Build history of the part. All positions in model axes, mm. Face numbers are marked on the shaded views. A direction names the side the tool comes from. Coordinates: 2 decimals unless noted, no trailing zeros. Order: outer loops, then holes, each group sorted by start corner. A loop starts at its lowest first (then second) coordinate and runs counter-clockwise, first axis right, second up. Notation, with made-up numbers: M 67.25,-35 L 120.25,-35 A23 cw 120.25,-21 Z; hole C -13.5,21 d11. An arc over 180 degrees is marked long. Write item = value, one per line. Start each with the question number.
Q1. Band-saw the part on D-D on z = 11.25. Write the cut outline in (x, y).
Q2. Band-saw the part on C-C on x = -4. Write the cut outline in (y, z).
Q3. Drill centre lines: probe 1 along Y at (x, z) = (-4, 0.6); probe 2 along Z at (x, y) = (2.5, 13); probe 3 along Y at (x, z) = (7, 15.5). Where is each one in solid material? Low to high.
Q4. Pin check, flat tips, straight feed: P1, Ø5, axis at x = -13, z = 17, coming from the +Y side; P2, Ø12, axis at x = 13.5, y = 10, coming from the +Z side. Stop position of each tip, or through.
Q5. Band-saw the part on A-A on y = -1.75. Write the cut outline in (x, z).
Q6. Band-saw the part on B-B on y = -12.75. Write the cut outline in (x, z).
Q7. 3-axis set-ups, long thin cutter, end or side, ignore diameter. For the marked faces 1 and 2: which of +Z, -Z, +X, -X, +Y, -Y reach the whole face in a straight line?
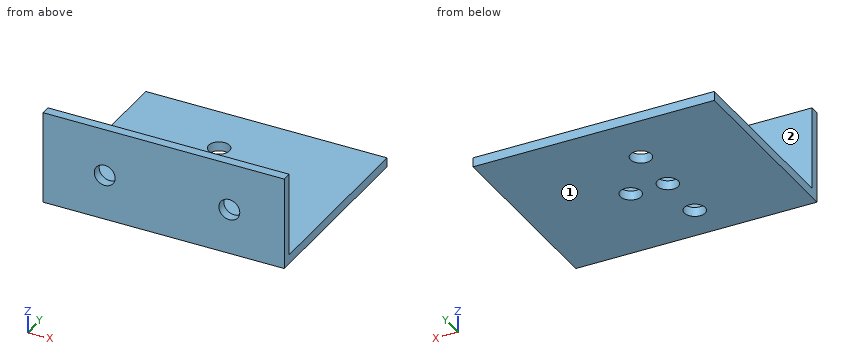
```python
from build123d import *

# Parameters (mm, degrees)
ESQUISSE1_W             = 52
ESQUISSE1_H             = 42
BOSS_EXTRU_1_DEPTH      = 20
ESQUISSE2_W             = 66.008627658
ESQUISSE2_H             = 40.946179855
ENL_V_MAT_EXTRU_1_DEPTH = 40
D_GAGEMENT_M41_D        = 4.5
D_GAGEMENT_M42_D        = 4.5


with BuildPart() as part:
    # Esquisse1 → Boss.-Extru.1 (new body)
    with BuildSketch(Plane.XY):
        Rectangle(ESQUISSE1_W, ESQUISSE1_H)
    extrude(amount=BOSS_EXTRU_1_DEPTH)

    # Esquisse2 → Enlèv. mat.-Extru.1 (cut)
    with BuildSketch(Plane(origin=(0, 21, 0), x_dir=(1, 0, 0), z_dir=(0, 1, 0))):
        with Locations((1.405901571, -22.473089928)):
            Rectangle(ESQUISSE2_W, ESQUISSE2_H)
    extrude(amount=-ENL_V_MAT_EXTRU_1_DEPTH, mode=Mode.SUBTRACT)

    # Dégagement M41 (through all)
    with Locations(Plane(origin=(0, 0, 0), x_dir=(-1, 0, 0), z_dir=(0, 0, -1))):
        with Locations((4, -12.75), (4, -1.75), (4, 9.25), (-4, -1.75)):
            Hole(D_GAGEMENT_M41_D / 2)

    # Dégagement M42 (through all)
    with Locations(Plane(origin=(0, -19, 0), x_dir=(1, 0, 0), z_dir=(0, 1, 0))):
        with Locations((-12.695679618, -9.785063319), (14.163037838, -9.785063319)):
            Hole(D_GAGEMENT_M42_D / 2)


solid = part.part
```
Recorded:
q1.outline = M -26,-21 L -14.4,-21 L -14.4,-19 L -26,-19 Z; M -10.99,-21 L 12.46,-21 L 12.46,-19 L -10.99,-19 Z; M 15.87,-21 L 26,-21 L 26,-19 L 15.87,-19 Z
q2.outline = M -21,0 L -15,0 L -15,2 L -19,2 L -19,20 L -21,20 Z; M -10.5,0 L -4,0 L -4,2 L -10.5,2 Z; M 0.5,0 L 7,0 L 7,2 L 0.5,2 Z; M 11.5,0 L 21,0 L 21,2 L 11.5,2 Z
q3.probe_1 = -21 to -15, -10.5 to -4, 0.5 to 7, 11.5 to 21
q3.probe_2 = 0 to 2
q3.probe_3 = -21 to -19
q4.P1 = -19
q4.P2 = 2
q5.outline = M -26,0 L -6.25,0 L -6.25,2 L -26,2 Z; M -1.75,0 L 1.75,0 L 1.75,2 L -1.75,2 Z; M 6.25,0 L 26,0 L 26,2 L 6.25,2 Z
q6.outline = M -26,0 L -6.25,0 L -6.25,2 L -26,2 Z; M -1.75,0 L 26,0 L 26,2 L -1.75,2 Z
q7.face_1 = -Z, +X, -X, +Y, -Y
q7.face_2 = +Z, +X, -X, +Y
